Solid Edge part; units mm, degrees
sketch "Sketch1" plane through (0, 0, 0) normal (0, -1, 0) x (1, 0, 0)
  circle A0 centre (-29.6968, 31.8389) radius 12.5
extrude "Protrusion1" add sketch "Sketch1" against normal blind 20
chamfer "Chamfer_1" distance 2 angle 45 1 edges at (-42.1968, 20, 31.8389)
sketch "Sketch2" plane through (-29.6968, 0, 31.8389) normal (0, -1, 0) x (1, 0, 0)
  circle A0 centre (0, 0) radius 14
  circle A1 centre (0, 0) radius 12
extrude "ExtrudedProtrusion_2" add sketch "Sketch2" along normal blind 2.5
fillet "Round_1" radius 1.5 1 edges at (-43.6968, -2.5, 31.8389)
sketch "Sketch3" plane through (-29.6968, 20, 31.8389) normal (0, 1, 0) x (1, 0, 0)
  circle A0 centre (7.5, 0) radius 1.25
  circle A1 centre (-7.5, 0) radius 1.25
extrude "ExtrudedProtrusion_3" add sketch "Sketch3" along normal blind 4
chamfer "Chamfer_2" distance 0.5 angle 45 2 edges at (-23.4468, 24, 31.8389) (-38.4468, 24, 31.8389)
sketch "Sketch4" plane through (-29.6968, 0, 31.8389) normal (0, -1, 0) x (-1, 0, 0)
  line L0 (-1.2639, 2) -> (-1.2639, -2)
  line L1 (-1.2639, -2) -> (-2.7639, -2)
  line L2 (-2.7639, -2) -> (-2.7639, 2)
  line L3 (-2.7639, 2) -> (-1.2639, 2)
  line L4 (-3.2639, 2) -> (-3.2639, -2)
  line L5 (-3.2639, -2) -> (-4.7639, -2)
  line L6 (-4.7639, -2) -> (-4.7639, 2)
  line L7 (-4.7639, 2) -> (-3.2639, 2)
  line L8 (-5.2639, 2) -> (-5.2639, -2)
  line L9 (-5.2639, -2) -> (-6.7639, -2)
  line L10 (-6.7639, -2) -> (-6.7639, 2)
  line L11 (-6.7639, 2) -> (-5.2639, 2)
  line L12 (2.75, 2) -> (2.75, -2)
  line L13 (2.75, -2) -> (1.25, -2)
  line L14 (1.25, -2) -> (1.25, 2)
  line L15 (1.25, 2) -> (2.75, 2)
  line L16 (4.75, 2) -> (4.75, -2)
  line L17 (4.75, -2) -> (3.25, -2)
  line L18 (3.25, -2) -> (3.25, 2)
  line L19 (3.25, 2) -> (4.75, 2)
  line L20 (6.75, 2) -> (6.75, -2)
  line L21 (6.75, -2) -> (5.25, -2)
  line L22 (5.25, -2) -> (5.25, 2)
  line L23 (5.25, 2) -> (6.75, 2)
  line L24 (-7.1233, 2) -> (-7.1233, -1.9996)
  line L25 (-7.1233, -1.9996) -> (-9.3891, 0)
  line L26 (-9.3891, 0) -> (-7.1233, 2)
  line L27 (7.1233, 2) -> (7.1233, -1.9996)
  line L28 (7.1233, -1.9996) -> (9.3891, 0)
  line L29 (9.3891, 0) -> (7.1233, 2)
  line L30 (0.75, 2) -> (0.75, -2)
  line L31 (0.75, -2) -> (-0.75, -2)
  line L32 (-0.75, -2) -> (-0.75, 2)
  line L33 (-0.75, 2) -> (0.75, 2)
  dimension "D1" = 0.75
  dimension "D2" = 0.75
extrude "ExtrudedProtrusion_4" add sketch "Sketch4" along normal blind 0.5
The listing builds one solid part. Answer for the finished solid, in the listing's coordinates (mm). A direction names the side the tool comes from. Round coordinates to 2 decimals unless told otherwise and drop trailing zeros. Loops run counter-clockwise (first coordinate to the right, second up) from the corner with the lowest first, then second, coordinate; pieces in that order, holes last.
Q1. Section A-A, the plane y = 21.5 is taken. Determine the outline of the cut face in (x, z).
Q2. Which of the six approach directions +Z, -Z, +X, -X, +Y, -Y give full straight-line access (tool end or side, diameter ignored) to faces 1 (the face through (-22, 24, 32)), 2 (the face through (-24, -0.5, 32)), 3 (the face through (-36, 21.7, 32.2))?
Q3. Find the intervals of material crossed by line 1 (Z direction, x = -29.25, y = 12); line 2 (Y direction, x = -29.5, z = 35); line 3 (X direction, y = 5.75, z = 32.25), in increasing order.
Q4. Section B-B, the plane y = 13 is taken. Determine the outline of the cut face in (x, z), then the cut area to 3 significant figures.
Q5. For a pull along Z with two mould halves and no side action, classify faces 4 (the face through (-32.298, -1.232, 43.554)), 5 (the face through (-19, -2.5, 38)), 6 (the face through (-37.969, -0.246, 30.853)), 7 (the face through (-21.042, 21.726, 31.36)) as released by +Z, released by -Z, zero draft, split by the parting line, or undercut.
Q6. Given pin 1 Ø10 at (x, y) = (-36, 11) entering from +Z; pin 2 Ø4 at (x, z) = (-24, 37.5) entering from -Y; pin 3 Ø2.5 at (x, z) = (-21.5, 32.5) entering from -Y, each flat-ended and moving along its own axis, determine where each tip first touches the part or whether it passes through.
Completed:
1. outline: circle Ø2.5 at (-37.2, 31.84); circle Ø2.5 at (-22.2, 31.84)
2. face 1: +Z, -Z, +X, -X, +Y
2. face 2: -Y
2. face 3: +Y
3. line 1: z = 19.35 to 44.33
3. line 2: y = 0 to 20
3. line 3: x = -42.19 to -17.2
4. outline: circle Ø25 at (-29.7, 31.84)
4. area: 491 mm2
5. face 4: undercut
5. face 5: zero draft
5. face 6: undercut
5. face 7: split by the parting line
6. pin 1: stops at z = 44.27
6. pin 2: stops at y = 0
6. pin 3: stops at y = -0.5
